```python
from build123d import *

# Parameters (mm, degrees)
F1_DEPTH = 2
F2_DEPTH = 2


with BuildPart() as f1:
    # F0 (on Top) → F1 (new body, symmetric)
    with BuildSketch(Plane.XY):
        with BuildLine():
            Line((0, 7.25), (0.1344755479, 4.2478719763))
            ThreePointArc((0.1344755479, 4.2478719763), (3.05237785, 2.957277373), (4.25, 0))
            Line((4.25, 0), (4.25, -2.5))
            Line((4.25, -2.5), (4.25, -5))
            ThreePointArc((4.25, -5), (3.5855613229, -7.2817208418), (1.8, -8.85))
            Line((1.8, -8.85), (1.8, -16.2))
            Line((1.8, -16.2), (10.1, -16.2))
            Line((10.1, -16.2), (11.2, -14.2))
            Line((11.2, -14.2), (10.1, -14.2))
            Line((10.1, -14.2), (10.1, -13))
            Line((10.1, -13), (14, -13))
            Line((14, -13), (14, -10))
            Line((14, -10), (7.25, -10))
            Line((7.25, -10), (7.25, -5))
            Line((7.25, -5), (7.25, -2.5))
            Line((7.25, -2.5), (7.25, 0))
            ThreePointArc((7.25, 0), (5.1265241636, 5.1265241636), (0, 7.25))
        make_face()
        with BuildLine():
            ThreePointArc((-3.5847754908, -0.3509463017), (-2.6563522123, 2.7015638934), (0.1344755479, 4.2478719763))
            Line((0.1344755479, 4.2478719763), (0, 7.25))
            ThreePointArc((0, 7.25), (-4.9161386256, 4.6766790635), (-6.5727609006, -0.6191685802))
            Line((-6.5727609006, -0.6191685802), (-6.3492423351, -3.1091564217))
            Line((-6.3492423351, -3.1091564217), (-6.1257237697, -5.5991442632))
            Line((-6.1257237697, -5.5991442632), (-5.6786866388, -10.5791199463))
            Line((-5.6786866388, -10.5791199463), (-12.4016538108, -11.182620073))
            Line((-12.4016538108, -11.182620073), (-12.1334315323, -14.1706054828))
            Line((-12.1334315323, -14.1706054828), (-8.2490504995, -13.8219165207))
            Line((-8.2490504995, -13.8219165207), (-8.1417615881, -15.0171106846))
            Line((-8.1417615881, -15.0171106846), (-9.2373562384, -15.1154588534))
            Line((-9.2373562384, -15.1154588534), (-7.9629467358, -17.0091009579))
            Line((-7.9629467358, -17.0091009579), (0.3038128981, -16.2670193205))
            Line((0.3038128981, -16.2670193205), (-0.3533316844, -8.9464550665))
            ThreePointArc((-0.3533316844, -8.9464550665), (-2.2719578811, -7.5440990943), (-3.1377383598, -5.3309219847))
            Line((-3.1377383598, -5.3309219847), (-3.3612569253, -2.8409341432))
            Line((-3.3612569253, -2.8409341432), (-3.5847754908, -0.3509463017))
        make_face()
    extrude(amount=F1_DEPTH, both=True)

    # F0 (on Top) → F2 (join)
    with BuildSketch(Plane.XY):
        with BuildLine():
            ThreePointArc((-0.7454173221, -2.3416861616), (-2.0552688347, 0.5327569072), (0.2019027868, 2.7425782149))
            Line((0.2019027868, 2.7425782149), (0.1344755479, 4.2478719763))
            ThreePointArc((0.1344755479, 4.2478719763), (-2.6563522123, 2.7015638934), (-3.5847754908, -0.3509463017))
            Line((-3.5847754908, -0.3509463017), (-3.3612569253, -2.8409341432))
            Line((-3.3612569253, -2.8409341432), (-3.1377383598, -5.3309219847))
            ThreePointArc((-3.1377383598, -5.3309219847), (-2.2719578811, -7.5440990943), (-0.3533316844, -8.9464550665))
            Line((-0.3533316844, -8.9464550665), (-0.5424341882, -6.8398607695))
            ThreePointArc((-0.5424341882, -6.8398607695), (-1.403238856, -5.0381101155), (-0.6700973051, -3.1807481254))
            Line((-0.6700973051, -3.1807481254), (-0.7454173221, -2.3416861616))
        make_face()
        with BuildLine():
            ThreePointArc((0.2019027868, 2.7425782149), (2.6476091797, 0.7434148448), (1.6, -2.2366269246))
            Line((1.6, -2.2366269246), (1.6, -3.0790627288))
            ThreePointArc((1.6, -3.0790627288), (2.4962673742, -4.8634379387), (1.8, -6.7349351573))
            Line((1.8, -6.7349351573), (1.8, -8.85))
            ThreePointArc((1.8, -8.85), (3.5855613229, -7.2817208418), (4.25, -5))
            Line((4.25, -5), (4.25, -2.5))
            Line((4.25, -2.5), (4.25, 0))
            ThreePointArc((4.25, 0), (3.05237785, 2.957277373), (0.1344755479, 4.2478719763))
            Line((0.1344755479, 4.2478719763), (0.2019027868, 2.7425782149))
        make_face()
    extrude(amount=F2_DEPTH)


solid = f1.part
```
For this review, take the finished solid that the model builds, in its own axes (mm). A direction names the side the tool comes from. Give positions to 0.01 mm unless a question says otherwise; leave off trailing zeros. Write each loop counter-clockwise with the first axis right and the second up, starting at its lowest first coordinate (ties: lowest second). Pieces come first, ordered by that corner, then holes. Notation, with made-up numbers: M 63.5,5.25 L 111.5,5.25 A29 cw 111.5,42.25 Z; hole C 52.25,50 d8. An arc over 180 degrees is marked long. Answer as CSV lines item,"result".
1. For pin 1 (1.2 mm diameter, centred on x = 4.5, z = -0.5, fed in from -Y); pin 2 (0.6 mm diameter, centred on y = -3.5, z = -0.5, fed in from -X); pin 3 (2.5 mm diameter, centred on x = 2, y = -3.5, fed in from -Z), all flat-tipped, find the tip position at first contact; note any pin that passes through.
Findings:
pin 1,"stops at y = -16.2"
pin 2,"stops at x = -6.34"
pin 3,"stops at z = 0"
2. Draft analysis for pull direction X (two halves, no side actions). For faces 1 (the cylindrical face through (-1.4, -5.1, 1)), 2 (the flat face through (11, -10, 0)), 3 (the flat face through (7.25, -5, 0)), state which applies: +X half, -X half, draft (parallel to the pull), parting line (faces both ways), or undercut.
Findings:
face 1,"undercut"
face 2,"draft"
face 3,"+X half"
3. For faces 4 (the flat face through (-0.707, -2.767, 0.986)), 5 (the cylindrical face through (3.02, 2.99, -0.99)), 6 (the flat face through (12, -13, 0)), 7 (the flat face through (6, -16.2, 0)), list the 3-axis set-ups (+Z, -Z, +X, -X, +Y, -Y) from which the entire face can be reached by the end or side of a thin tool; tool diameter is ignored.
Findings:
face 4,"+Z, -Z"
face 5,"-Z"
face 6,"+Z, -Z, +X"
face 7,"+Z, -Z, +X, -Y"
4. Consider section C-C, the plane x = 10.5. Write out the cut boundary in (y, z), then the cut area to 3 significant figures.
Findings:
outline,"M -15.47,-2 L -14.2,-2 L -14.2,2 L -15.47,2 Z; M -13,-2 L -10,-2 L -10,2 L -13,2 Z"
area,"17.1 mm2"
5. Consider section A-A, the plane y = 1.75. Write out the cut boundary in (x, z), then the cut area to 3 significant figures.
Findings:
outline,"M -6.39,-2 L -3.24,-2 L -3.24,0 L -1.5,0 L -1.5,2 L -6.39,2 Z; M 2.12,0 L 3.87,0 L 3.87,-2 L 7.04,-2 L 7.04,2 L 2.12,2 Z"
area,"32.3 mm2"
6. Consider section B-B, the plane z = 1.55. Write out the cut boundary in (x, y), then the cut area to 3 significant figures.
Findings:
outline,"M -12.4,-11.18 L -12.13,-14.17 L -8.25,-13.82 L -8.14,-15.02 L -9.24,-15.12 L -7.96,-17.01 L 0.3,-16.27 L -0.54,-6.84 A2.5 cw -0.67,-3.18 L -0.75,-2.34 A2.75 cw 0.2,2.74 A2.75 cw 1.6,-2.24 L 1.6,-3.08 A2.5 cw 1.8,-6.73 L 1.8,-16.2 L 10.1,-16.2 L 11.2,-14.2 L 10.1,-14.2 L 10.1,-13 L 14,-13 L 14,-10 L 7.25,-10 L 7.25,0 A7.25 ccw 0,7.25 A7.25 ccw -6.57,-0.62 L -5.68,-10.58 Z"
area,"302 mm2"
7. Wall thickness on line 1 (Y direction, x = 11.25, z = 0.9); line 2 (X direction, y = -9, z = -1.2); line 3 (X direction, y = -11.75, z = 1.2): over which ranges is each line inside the solid? List them lowest first.
Findings:
line 1,"y = -13 to -10"
line 2,"x = -5.82 to -0.35, 1.8 to 7.25"
line 3,"x = -12.35 to -0.1, 1.8 to 14"
8. Consider section D-D, the plane z = -1. Write out the cut boundary in (x, y).
Findings:
outline,"M -12.4,-11.18 L -12.13,-14.17 L -8.25,-13.82 L -8.14,-15.02 L -9.24,-15.12 L -7.96,-17.01 L 0.3,-16.27 L -0.35,-8.95 A4.25 cw -3.14,-5.33 L -3.58,-0.35 A4.25 cw 0.13,4.25 A4.25 cw 4.25,0 L 4.25,-5 A4.25 cw 1.8,-8.85 L 1.8,-16.2 L 10.1,-16.2 L 11.2,-14.2 L 10.1,-14.2 L 10.1,-13 L 14,-13 L 14,-10 L 7.25,-10 L 7.25,0 A7.25 ccw 0,7.25 A7.25 ccw -6.57,-0.62 L -5.68,-10.58 Z"
